Check sheet for the modelled part. Datum: model origin and axes. Units: mm. A direction names the side the tool comes from. Round coordinates to 2 decimals unless told otherwise and drop trailing zeros. Write each loop counter-clockwise with the first axis right and the second up, starting at its lowest first coordinate (ties: lowest second). Pieces come first, ordered by that corner, then holes.
Item 1: Cross-section at A-A on z = 2.75. Enter the section's corners in (x, y).
Item 2: Release check for a two-part mould opening along Y. For faces 5 (the flat face through (99, 23, 5.01)), 6 (the flat face through (47, -115.098, 2)), 7 (the flat face through (35, -95.5, 2)) record: +Y half, -Y half, draft (parallel to the pull), parting line (faces both ways), or undercut.
Item 3: Tool access check on faces 1 (the flat face through (84, -105.098, 3)), 2 (the flat face through (5, -22, 3)), 3 (the flat face through (24, -25, 2)), 4 (the flat face through (93, -44, 5)). Record the directions out of +Z, -Z, +X, -X, +Y, -Y that give a thin tool (end or side, any length) a straight path to the whole face; none if there is none.
Item 4: Material ranges on line 1 (Z direction, x = 71.5, y = -23); line 2 (X direction, y = -16, z = 0.9); line 3 (Y direction, x = 91, z = 0.9), recorded low to high.
Item 5: Cross-section at C-C on y = -77. Enter the section's corners in (x, z).
Item 6: Go/stop test with flat-tipped pins: pin 1 Ø3 at (x, y) = (102.5, -87.5) entering from +Z; pin 2 Ø1.5 at (x, z) = (19.5, 2) entering from -Y; pin 3 Ø2.5 at (y, z) = (-107, 3.5) entering from +X. Record where each tip stops, or that it passes through.
from build123d import *

# Parameters (mm, degrees)
BOSS_EXTRU_1_DEPTH      = 5
BOSS_EXTRU_2_DEPTH      = 0.01
ESQUISSE3_W             = 10
ESQUISSE3_H             = 3
ENL_V_MAT_EXTRU_1_DEPTH = 231.967242256
ENL_V_MAT_EXTRU_2_DEPTH = 231.967242256


with BuildPart() as part:
    # Esquisse1 → Boss.-Extru.1 (new body)
    with BuildSketch(Plane.XY):
        with BuildLine():
            Line((0, 0), (0, -25))
            Line((0, -25), (37.5, -25))
            Line((37.5, -25), (37.5, -95.5))
            Line((37.5, -95.5), (32.5, -95.5))
            Line((32.5, -95.5), (36.487358688, -115.098494092))
            Line((36.487358688, -115.098494092), (88.487358688, -115.098494092))
            Line((88.487358688, -115.098494092), (159.198036807, -44.387815974))
            ThreePointArc((159.198036807, -44.387815974), (187.146342861, -3.044299659), (200.182925478, 45.126663235))
            Line((200.182925478, 45.126663235), (43.682925478, 43.998857528))
            ThreePointArc((43.682925478, 43.998857528), (12.775400091, 31.000392909), (0, 0))
        make_face()
    extrude(amount=BOSS_EXTRU_1_DEPTH)

    # Esquisse2 → Boss.-Extru.2 (add)
    with BuildSketch(Plane.XY.offset(5)):
        with BuildLine():
            Line((0, 0), (188.5, 0))
            ThreePointArc((188.5, 0), (195.764398976, 22.194945018), (200.182925478, 45.126663235))
            Line((200.182925478, 45.126663235), (43.682925478, 43.998857528))
            ThreePointArc((43.682925478, 43.998857528), (12.775400091, 31.000392909), (0, 0))
        make_face()
    extrude(amount=BOSS_EXTRU_2_DEPTH)

    # Esquisse3 → Enlèv. mat.-Extru.1 (cut, through all)
    with BuildSketch(Plane.XY.offset(5)):
        with Locations((5, -23.5)):
            Rectangle(ESQUISSE3_W, ESQUISSE3_H)
    extrude(amount=-ENL_V_MAT_EXTRU_1_DEPTH, mode=Mode.SUBTRACT)

    # Esquisse4 → Enlèv. mat.-Extru.2 (cut, through all)
    with BuildSketch(Plane.XY.offset(5)):
        Polygon((88.487358688, -105.098494092), (68.487358688, -105.098494092), (68.487358688, -111.098494092), (58.487358688, -115.098494092), (68.487358688, -115.098494092), (88.487358688, -115.098494092), (98.487358688, -105.098494092), align=None)
    extrude(amount=-ENL_V_MAT_EXTRU_2_DEPTH, mode=Mode.SUBTRACT)


solid = part.part
Response values:
1. outline: (0, -22) - (10, -22) - (10, -25) - (37.5, -25) - (37.5, -95.5) - (32.5, -95.5) - (36.49, -115.1) - (58.49, -115.1) - (68.49, -111.1) - (68.49, -105.1) - (98.49, -105.1) - (159.2, -44.39) arc R151.85 ccw to (200.18, 45.13) - (43.68, 44) arc R44 ccw to (0, 0) - close
2. face 5: draft
2. face 6: -Y half
2. face 7: undercut
3. face 1: +Z, -Z, +X, -Y
3. face 2: +Z, -Z, -X, -Y
3. face 3: +Z, -Z, -X
3. face 4: +Z, +X, -X, +Y, -Y
4. line 1: z = 0 to 5
4. line 2: x = 0 to 180.44
4. line 3: y = -105.1 to 44.34
5. outline: (37.5, 0) - (126.59, 0) - (126.59, 5) - (37.5, 5) - close
6. pin 1: stops at z = 5
6. pin 2: stops at y = -25
6. pin 3: stops at x = 68.49
